Here's how the part is built. I have some questions about the finished solid (model axes, mm). A direction names the side the tool comes from. Coordinates: 2 decimals unless noted, no trailing zeros. Order: outer loops, then holes, each group sorted by start corner. A loop starts at its lowest first (then second) coordinate and runs counter-clockwise, first axis right, second up. Notation, with made-up numbers: (9.5, 48) - (41.5, 48) arc R10 cw to (41.5, 52) - close; hole circle Ø3 at (25.5, 84). An arc over 180 degrees is marked (long way). Answer as CSV lines item,"result". Start each with the question number.
Q1. Thinking about a two-plate mould opening in Z: for faces 1 (the face through (0, -3, 25)), 2 (the face through (-3, 0, 30)), 3 (the face through (-1.14, -1.94, 12.32)), which applies, released by +Z, released by -Z, zero draft, split by the parting line, or undercut?
Q2. Suppose I cut it at B-B (z = 4). Please give me the cut outline in (x, y), then the cut area to 3 significant figures.
Q3. For faces 4 (the face through (2.25, 0, 15)), 5 (the face through (3, -2.309, 27)), 6 (the face through (0, 3, 25)), 7 (the face through (3, 2.309, 27)), 8 (the face through (1.97, 3.48, 11.69)), which set-ups out of +Z, -Z, +X, -X, +Y, -Y let a thin tool reach every point of the face, with its end or its side?
Q4. Suppose I cut it at C-C (x = -3). Please give me the cut outline in (y, z), then the cut area to 3 significant figures.
Q5. Suppose I cut it at A-A (y = 0). Please give me the cut outline in (x, z), then the cut area to 3 significant figures.
Q6. I need wall thicknesses on line 1 (Y direction, x = -3.1, z = 29); line 2 (X direction, y = -0.25, z = 21.5); line 3 (Z direction, x = 0.5, y = -2.5). Which ranges of each line are inside material? Lowest first, please.
Q7. For pin 1 Ø1 at (x, y) = (0, 3) entering from +Z; pin 2 Ø3 at (x, y) = (0, 0) entering from +Z; pin 3 Ø1.9 at (x, z) = (-3.5, 27.5) entering from -Y; pin 4 Ø1.8 at (y, z) = (0, 29) entering from +X, each with a flat end and sliding along its axis, tell me the tip position at first contact or that it passes through.
Q8. Suppose I cut it at D-D (y = 2). Please give me the cut outline in (x, z).
from build123d import *

# Parameters (mm, degrees)
EXTRUDE_1_DEPTH = 25
SKETCH_2_R      = 1.25
EXTRUDE_2_DEPTH = 2
SKETCH_3_R      = 1
EXTRUDE_3_DEPTH = 1.75
SKETCH_4_R      = 1
EXTRUDE_4_DEPTH = 1.75


with BuildPart() as part:
    # 스케치1 → 보스-돌출1 (new body)
    with BuildSketch(Plane.XY):
        Polygon((0, 4.618802154), (-4, 2.309401077), (-4, -2.309401077), (0, -4.618802154), (4, -2.309401077), (4, 2.309401077), align=None)
        Polygon((0, 2.598076211), (-2.25, 1.299038106), (-2.25, -1.299038106), (0, -2.598076211), (2.25, -1.299038106), (2.25, 1.299038106), align=None, mode=Mode.SUBTRACT)
    extrude(amount=EXTRUDE_1_DEPTH)

    # 스케치2 → 보스-돌출2 (add)
    with BuildSketch(Plane(origin=(0, 0, 0), x_dir=(-1, 0, 0), z_dir=(0, 0, -1))):
        Polygon((0, 4.618802154), (-4, 2.309401077), (-4, -2.309401077), (0, -4.618802154), (4, -2.309401077), (4, 2.309401077), align=None)
        Circle(SKETCH_2_R, mode=Mode.SUBTRACT)
    extrude(amount=EXTRUDE_2_DEPTH)

    # 스케치3 → 보스-돌출3 (add)
    with BuildSketch(Plane.ZY.offset(4)):
        with BuildLine():
            Line((25, 2.309401077), (29, 2.309401077))
            ThreePointArc((29, 2.309401077), (31.309401077, 0), (29, -2.309401077))
            Line((29, -2.309401077), (25, -2.309401077))
            Line((25, -2.309401077), (25, 2.309401077))
        make_face()
        with Locations((29, 0)):
            Circle(SKETCH_3_R, mode=Mode.SUBTRACT)
    extrude(amount=-EXTRUDE_3_DEPTH)

    # 스케치4 → 보스-돌출4 (add)
    with BuildSketch(Plane(origin=(4, 0, 0), x_dir=(0, 0, -1), z_dir=(1, 0, 0))):
        with BuildLine():
            Line((-29, 2.309401077), (-25, 2.309401077))
            Line((-25, 2.309401077), (-25, -2.309401077))
            Line((-25, -2.309401077), (-29, -2.309401077))
            ThreePointArc((-29, -2.309401077), (-31.309401077, 0), (-29, 2.309401077))
        make_face()
        with Locations((-29, 0)):
            Circle(SKETCH_4_R, mode=Mode.SUBTRACT)
    extrude(amount=-EXTRUDE_4_DEPTH)


solid = part.part
Here are the results:
1,face 1,"released by +Z"
1,face 2,"undercut"
1,face 3,"zero draft"
2,outline,"(-4, -2.31) - (0, -4.62) - (4, -2.31) - (4, 2.31) - (0, 4.62) - (-4, 2.31) - close; hole (-2.25, -1.3) - (0, -2.6) - (2.25, -1.3) - (2.25, 1.3) - (0, 2.6) - (-2.25, 1.3) - close"
2,area,"37.9 mm²"
3,face 4,"+Z"
3,face 5,"+Z, +X, -X, -Y"
3,face 6,"+Z, +Y"
3,face 7,"+Z, +X, -X, +Y"
3,face 8,"+Z, -Z, +X, +Y"
4,outline,"(-2.89, -2) - (2.89, -2) - (2.89, 25) - (2.31, 25) - (2.31, 29) arc R2.31 ccw to (-2.31, 29) - (-2.31, 25) - (-2.89, 25) - close; hole circle Ø2 at (0, 29)"
4,area,"180 mm²"
5,outline,"(-4, -2) - (-1.25, -2) - (-1.25, 0) - (-2.25, 0) - (-2.25, 28) - (-4, 28) - close; (-4, 30) - (-2.25, 30) - (-2.25, 31.31) - (-4, 31.31) - close; (1.25, -2) - (4, -2) - (4, 28) - (2.25, 28) - (2.25, 0) - (1.25, 0) - close; (2.25, 30) - (4, 30) - (4, 31.31) - (2.25, 31.31) - close"
5,area,"114 mm²"
6,line 1,"y = -2.31 to -1, 1 to 2.31"
6,line 2,"x = -4 to -2.25, 2.25 to 4"
6,line 3,"z = -2 to 25"
7,pin 1,"stops at z = 25"
7,pin 2,"stops at z = 0"
7,pin 3,"stops at y = -2.31"
7,pin 4,"passes through"
8,outline,"(-4, -2) - (4, -2) - (4, 30.15) - (2.25, 30.15) - (2.25, 25) - (1.04, 25) - (1.04, 0) - (-1.04, 0) - (-1.04, 25) - (-2.25, 25) - (-2.25, 30.15) - (-4, 30.15) - close"
